```python
from build123d import *

# Parameters (mm, degrees)
F0_W     = 24
F0_H     = 24
F0_R     = 1.35
F0_R_2   = 1.9
F1_DEPTH = 8
F2_W     = 8.4
F2_H     = 16.8
F2_R     = 1.9
F3_DEPTH = 5
F2_W_2   = 11
F2_H_2   = 18.5
F4_DEPTH = 2.9
F5_R     = 4


with BuildPart() as f1:
    # F0 (on Top) → F1 (new body)
    with BuildSketch(Plane.XY):
        Rectangle(F0_W, F0_H)
        with Locations((-8, -8)):
            Circle(F0_R, mode=Mode.SUBTRACT)
        with Locations((8, -8)):
            Circle(F0_R, mode=Mode.SUBTRACT)
        with Locations((0, -3)):
            Circle(F0_R_2, mode=Mode.SUBTRACT)
        with Locations((-8, 8)):
            Circle(F0_R, mode=Mode.SUBTRACT)
        with Locations((0, 3)):
            Circle(F0_R_2, mode=Mode.SUBTRACT)
        with Locations((8, 8)):
            Circle(F0_R, mode=Mode.SUBTRACT)
    extrude(amount=F1_DEPTH)

    # F2 (on face) → F3 (cut)
    with BuildSketch(Plane.XY.offset(8)):
        Rectangle(F2_W, F2_H)
        with Locations((0, -3)):
            Circle(F2_R, mode=Mode.SUBTRACT)
        with Locations((0, 3)):
            Circle(F2_R, mode=Mode.SUBTRACT)
    extrude(amount=-F3_DEPTH, mode=Mode.SUBTRACT)

    # F2 (on face) → F4 (cut)
    with BuildSketch(Plane.XY.offset(8)):
        Rectangle(F2_W_2, F2_H_2)
        Rectangle(F2_W, F2_H, mode=Mode.SUBTRACT)
    extrude(amount=-F4_DEPTH, mode=Mode.SUBTRACT)

    # F5
    f5_edges = [f1.edges().sort_by_distance(p)[0] for p in [
        (-12, 12, 4),
        (12, 12, 4),
        (12, -12, 4),
        (-12, -12, 4),
    ]]
    fillet(f5_edges, radius=F5_R)


solid = f1.part
```
CAD build for the part. Positions are in the model's coordinates, mm. A direction names the side the tool comes from. Round coordinates to 2 decimals unless told otherwise and drop trailing zeros. Write each loop counter-clockwise with the first axis right and the second up, starting at its lowest first coordinate (ties: lowest second). Pieces come first, ordered by that corner, then holes. Notation, with made-up numbers: (50, 30.5) - (99, 30.5) arc R24 ccw to (99, 52.5) - close; hole circle Ø2 at (74, -16). An arc over 180 degrees is marked (long way). Return JSON: item names as keys, results as strings. Group by question number.
Item 1: Probe probe 1 along Y at (x, z) = (0, 1.6); probe 2 along Y at (x, z) = (8, 1.5); probe 3 along Y at (x, z) = (0.5, 6.25). List the from-to ranges inside material, lowest first.
Item 2: Band-saw the part on C-C on x = 0. List the corners of the cut face in (y, z), plus the area to 3 significant figures.
Item 3: Mould opens along Y. For faces 1 (the face through (-0.247, -1.116, 1.479)), 2 (the face through (-6, 0, 8)), 3 (the face through (10.797, -10.859, 4.056)) say: +Y half, -Y half, draft (parallel to the pull), parting line (faces both ways), or undercut.
Item 4: Band-saw the part on B-B on z = 6.5. List the corners of the cut face in (x, y), plus the area to 3 significant figures.
Item 5: Band-saw the part on D-D on x = -3.5. List the corners of the cut face in (y, z).
Item 6: 3-axis set-ups, long thin cutter, end or side, ignore diameter. For faces 4 (the face through (4.2, 0, 4)), 5 (the face through (0, 12, 4)): which of +Z, -Z, +X, -X, +Y, -Y reach the whole face in a straight line?
Item 7: Band-saw the part on A-A on y = 3. List the corners of the cut face in (x, z), plus the area to 3 significant figures.
Item 8: Flat gauge pins, fed straight in: pin 1 Ø2 at (x, y) = (-8, -8) entering from +Z; pin 2 Ø10 at (x, y) = (-4, -5) entering from -Z; pin 3 Ø5 at (x, y) = (0, -3.5) entering from +Z; pin 4 Ø5 at (x, y) = (2, 3.5) entering from +Z. Where does each tip first touch, or does it go through?
Resolved:
{
 "1": {"probe 1": "y = -12 to -4.9, -1.1 to 1.1, 4.9 to 12", "probe 2": "y = -12 to -9.35, -6.65 to 6.65, 9.35 to 12", "probe 3": "y = -12 to -9.25, 9.25 to 12"},
 "2": {"outline": "(-12, 0) - (-4.9, 0) - (-4.9, 3) - (-8.4, 3) - (-8.4, 5.1) - (-9.25, 5.1) - (-9.25, 8) - (-12, 8) - close; (-1.1, 0) - (1.1, 0) - (1.1, 3) - (-1.1, 3) - close; (4.9, 0) - (12, 0) - (12, 8) - (9.25, 8) - (9.25, 5.1) - (8.4, 5.1) - (8.4, 3) - (4.9, 3) - close", "area": "80.3 mm²"},
 "3": {"face 1": "undercut", "face 2": "draft", "face 3": "-Y half"},
 "4": {"outline": "(-12, -8) arc R4 ccw to (-8, -12) - (8, -12) arc R4 ccw to (12, -8) - (12, 8) arc R4 ccw to (8, 12) - (-8, 12) arc R4 ccw to (-12, 8) - close; hole circle Ø2.7 at (-8, -8); hole circle Ø2.7 at (-8, 8); hole (-5.5, -9.25) - (5.5, -9.25) - (5.5, 9.25) - (-5.5, 9.25) - close; hole circle Ø2.7 at (8, -8); hole circle Ø2.7 at (8, 8)", "area": "336 mm²"},
 "5": {"outline": "(-12, 0) - (12, 0) - (12, 8) - (9.25, 8) - (9.25, 5.1) - (8.4, 5.1) - (8.4, 3) - (-8.4, 3) - (-8.4, 5.1) - (-9.25, 5.1) - (-9.25, 8) - (-12, 8) - close"},
 "6": {"face 4": "+Z", "face 5": "+Z, -Z, +X, -X, +Y"},
 "7": {"outline": "(-12, 0) - (-1.9, 0) - (-1.9, 3) - (-4.2, 3) - (-4.2, 5.1) - (-5.5, 5.1) - (-5.5, 8) - (-12, 8) - close; (1.9, 0) - (12, 0) - (12, 8) - (5.5, 8) - (5.5, 5.1) - (4.2, 5.1) - (4.2, 3) - (1.9, 3) - close", "area": "131 mm²"},
 "8": {"pin 1": "passes through", "pin 2": "stops at z = 0", "pin 3": "stops at z = 3", "pin 4": "stops at z = 5.1"}
}
